Source: CAD feature listing. Evaluate the final solid. Frame: model axes, mm. A direction names the side the tool comes from. Coordinates: 2 decimals unless noted, no trailing zeros. Loops run counter-clockwise (first coordinate to the right, second up) from the corner with the lowest first, then second, coordinate; pieces in that order, holes last. Notation, with made-up numbers: (-6, 33) -> (35, 33) arc R21 ccw to (35, 67) -> close; hole circle Ø3 at (54, 25). An arc over 180 degrees is marked (long way). Answer as CSV lines item,"result".
from build123d import *

# Parameters (mm, degrees)
F1_W     = 34
F1_H     = 69
F1_W_2   = 30
F1_H_2   = 65
F2_DEPTH = 8
F3_DEPTH = 2
F4_R     = 3
F5_W     = 27.269229
F5_H     = 1.5
F6_DEPTH = 25
F7_DEPTH = 45.4


with BuildPart() as f2:
    # F1 (on face) → F2 (new body)
    with BuildSketch(Plane.XY):
        with Locations((1.3335, 11.379073)):
            Rectangle(F1_W, F1_H)
        with Locations((1.3335, 11.379073)):
            Rectangle(F1_W_2, F1_H_2, mode=Mode.SUBTRACT)
    extrude(amount=F2_DEPTH)

    # F1 (on face) → F3 (join)
    with BuildSketch(Plane.XY):
        with Locations((1.3335, 11.379073)):
            Rectangle(F1_W, F1_H)
    extrude(amount=F3_DEPTH)

    # F4
    f4_edges = [f2.edges().sort_by_distance(p)[0] for p in [
        (-15.6665, 45.879073, 4),
        (18.3335, 45.879073, 4),
        (18.3335, -23.120927, 4),
        (-15.6665, -23.120927, 4),
        (-13.6665, 43.879073, 5),
        (16.3335, 43.879073, 5),
        (16.3335, -21.120927, 5),
        (-13.6665, -21.120927, 5),
    ]]
    fillet(f4_edges, radius=F4_R)

    # F5 (on Front) → F6 (cut)
    with BuildSketch(Plane.XZ):
        with Locations((1.363065, 6.764378)):
            Rectangle(F5_W, F5_H)
    extrude(amount=F6_DEPTH, mode=Mode.SUBTRACT)

    # F5 (on Front) → F7 (cut)
    with BuildSketch(Plane.XZ):
        with Locations((1.363065, 6.764378)):
            Rectangle(F5_W, F5_H)
    extrude(amount=-F7_DEPTH, mode=Mode.SUBTRACT)


solid = f2.part
(1) Cut plane A-A (z = 5). Return the cut outline in (x, y), then the cut area to 3 significant figures.
Computed values:
outline,"(-15.67, -20.12) arc R3 ccw to (-12.67, -23.12) -> (15.33, -23.12) arc R3 ccw to (18.33, -20.12) -> (18.33, 42.88) arc R3 ccw to (15.33, 45.88) -> (-12.67, 45.88) arc R3 ccw to (-15.67, 42.88) -> close; hole (-13.67, -18.12) arc R3 ccw to (-10.67, -21.12) -> (13.33, -21.12) arc R3 ccw to (16.33, -18.12) -> (16.33, 40.88) arc R3 ccw to (13.33, 43.88) -> (-10.67, 43.88) arc R3 ccw to (-13.67, 40.88) -> close"
area,"396 mm^2"
(2) Cut plane B-B (x = 12). Return the cut outline in (y, z).
Computed values:
outline,"(-23.12, 0) -> (45.88, 0) -> (45.88, 8) -> (43.88, 8) -> (43.88, 7.51) -> (45.4, 7.51) -> (45.4, 6.01) -> (43.88, 6.01) -> (43.88, 2) -> (-21.12, 2) -> (-21.12, 6.01) -> (-23.12, 6.01) -> close; (-23.12, 7.51) -> (-21.12, 7.51) -> (-21.12, 8) -> (-23.12, 8) -> close"
(3) Access query for faces 1 (the flat face through (1, -23.121, 3)), 2 (the flat face through (1, 45, 6.014)), 3 (the flat face through (16.334, 11, 5)). Directions: +Z, -Z, +X, -X, +Y, -Y. A direction counts if a zero-diameter tool reaches every point of the face in a straight line with its end or side. Return the directions, or none.
Computed values:
face 1,"+Z, -Z, +X, -X, -Y"
face 2,"-Y"
face 3,"+Z"
(4) Cut plane C-C (y = -17.5). Return the cut outline in (x, z), then the cut area to 3 significant figures.
Computed values:
outline,"(-15.67, 0) -> (18.33, 0) -> (18.33, 8) -> (16.33, 8) -> (16.33, 2) -> (-13.67, 2) -> (-13.67, 8) -> (-15.67, 8) -> close"
area,"92.0 mm^2"
(5) Draft query along Y for faces 4 (the cylindrical face through (15.478, -20.219, 5.042)), 5 (the flat face through (14.998, -22, 7)), 6 (the cylindrical face through (-14.81, -22.22, 4.06)). Return one class per face: released by +Y, released by -Y, zero draft, split by the parting line, or undercut.
Computed values:
face 4,"undercut"
face 5,"zero draft"
face 6,"released by -Y"
(6) Pin query (flat end, axial travel): pin 1 Ø5 at (x, y) = (-5.5, 31.5) entering from +Z; pin 2 Ø0.5 at (y, z) = (-22, 7) entering from -X; pin 3 Ø1.2 at (y, z) = (-22.5, 7) entering from +X. Return the tip coordinate at first contact, or that it passes through.
Computed values:
pin 1,"z = 2"
pin 2,"x = -15.19"
pin 3,"x = 17.75"
(7) Material intervals for L1, parallel to Y at x = 9, z = 3.75; L2, parallel to Y at x = 15, z = 5.75; L3, parallel to X at y = 30, z = 2.5, sorted ascending. Write a range as [from, to].
Computed values:
L1,"[-23.12, -21.12], [43.88, 45.88]"
L2,"[-23.12, -20.62], [43.37, 45.88]"
L3,"[-15.67, -13.67], [16.33, 18.33]"
